CAD build for the part. Positions are in the model's coordinates, mm. Face numbers are marked on the shaded views. A direction names the side the tool comes from. Round coordinates to 2 decimals unless told otherwise and drop trailing zeros. Loops run counter-clockwise (first coordinate to the right, second up) from the corner with the lowest first, then second, coordinate; pieces in that order, holes last. Notation, with made-up numbers: M -9,27 L 5,27 A19 cw 5,41 Z; hole C 7.5,38.5 d3. An arc over 180 degrees is marked long. Use one line per item in the form item = value.
Autodesk Inventor part; units mm, degrees
ref_plane "h1_XY" through (-96.0374, 0, 0) normal (0, 1, 0) x (1, 0, 0)
ref_plane "h1_YZ" through (-96.0374, 0, 0) normal (1, 0, 0) x (0, 0, -1)
ref_plane "h1_ZX" through (-96.0374, 0, 0) normal (0, 0, -1) x (0, 1, 0)
sketch "Sketch_3" plane through (0, 0, 0) normal (0, 0, 1) x (1, 0, 0)
  line L0 (0, 0) -> (-96.0374, 0)
  line L1 (-96.0374, 0) -> (-96.0374, 1.9406)
  line L2 (-96.0374, 1.9406) -> (-95.565, 2.413)
  line L3 (-95.565, 2.413) -> (0, 2.413)
  line L4 (0, 2.413) -> (0, 0)
  line L5 (0, 0) -> (-96.0374, 0)
revolve "Revolution1" add sketch "Sketch_3" angle 360 about axis through (0, 0, 0) along (1, 0, 0)
thread "Thread1"
sketch "Sketch_17" plane through (0, 0, 0) normal (0, 0, 1) x (1, 0, 0)
  line L0 (96.0374, 0) -> (-96.0374, 0)
  line L1 (-83.5914, 2.413) -> (-83.5914, 2.159)
  line L2 (-83.5914, 2.159) -> (-83.3374, 2.159)
  line L3 (-83.3374, 2.159) -> (-83.3374, 2.413)
  line L4 (-83.3374, 2.413) -> (-83.5914, 2.413)
revolve "Revolution2" cut sketch "Sketch_17" angle 360 about axis through (96.0374, 0, 0) along (1, 0, 0)
sketch "Sketch_12" plane through (0, 0, 0) normal (0, 0, 1) x (1, 0, 0)
  line L0 (1.524, 0) -> (-15.875, 0)
  line L1 (-15.875, 0) -> (-15.875, 7.2771)
  line L2 (-15.875, 7.2771) -> (1.524, 7.2771)
  line L3 (1.524, 7.2771) -> (1.524, 0)
  line L4 (1.524, 0) -> (-15.875, 0)
revolve "Revolution3" add sketch "Sketch_12" angle 360 about axis through (1.524, 0, 0) along (1, 0, 0)
ref_plane "h1_XY" through (-96.0374, 0, 0) normal (0, 1, 0) x (1, 0, 0)
ref_plane "h1_YZ" through (-96.0374, 0, 0) normal (1, 0, 0) x (0, 0, -1)
ref_plane "h1_ZX" through (-96.0374, 0, 0) normal (0, 0, -1) x (0, 1, 0)
ref_plane "h2_XY" through (-83.3374, 0, 0) normal (0, 1, 0) x (1, 0, 0)
ref_plane "h2_YZ" through (-83.3374, 0, 0) normal (1, 0, 0) x (0, 0, -1)
ref_plane "h2_ZX" through (-83.3374, 0, 0) normal (0, 0, -1) x (0, 1, 0)
ref_plane "k1_XY" through (-96.0374, 0, -2.413) normal (0, 1, 0) x (1, 0, 0)
ref_plane "k1_YZ" through (-96.0374, 0, -2.413) normal (1, 0, 0) x (0, 0, -1)
ref_plane "k1_ZX" through (-96.0374, 0, -2.413) normal (0, 0, -1) x (0, 1, 0)
ref_plane "k2_XY" through (-96.0374, 0, 2.413) normal (0, 1, 0) x (1, 0, 0)
ref_plane "k2_YZ" through (-96.0374, 0, 2.413) normal (1, 0, 0) x (0, 0, -1)
ref_plane "k2_ZX" through (-96.0374, 0, 2.413) normal (0, 0, -1) x (0, 1, 0)
ref_plane "start_XY" through (-83.3374, 0, 0) normal (0, 1, 0) x (1, 0, 0)
ref_plane "start_YZ" through (-83.3374, 0, 0) normal (1, 0, 0) x (0, 0, -1)
ref_plane "start_ZX" through (-83.3374, 0, 0) normal (0, 0, -1) x (0, 1, 0)
ref_plane "to_prc_XY" through (-83.3374, 0, 0) normal (1, 0, 0) x (0, 0, -1)
ref_plane "to_prc_YZ" through (-83.3374, 0, 0) normal (0, 0, -1) x (0, 1, 0)
ref_plane "to_prc_ZX" through (-83.3374, 0, 0) normal (0, 1, 0) x (1, 0, 0)
ref_plane "to_rod_guide_XY" through (-96.0374, 0, 0) normal (1, 0, 0) x (0, 0, -1)
ref_plane "to_rod_guide_YZ" through (-96.0374, 0, 0) normal (0, 0, -1) x (0, 1, 0)
ref_plane "to_rod_guide_ZX" through (-96.0374, 0, 0) normal (0, 1, 0) x (1, 0, 0)
properties part number "D-75081.25-0.25XP-3.781-3pos" material "Steel"
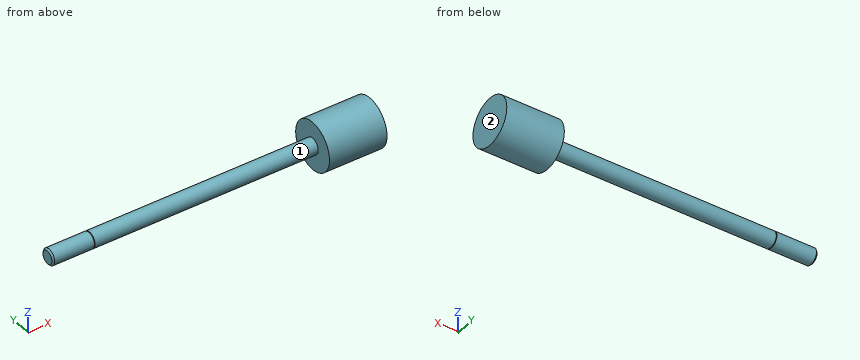
1. Cut at C-C on x = -49.5. Write the cut outline in (y, z), and give its area (3 significant figures).
Completed:
outline = C 0,0 d4.83
area = 18.3 mm2
2. Drop flat-ended pins along their axis: P1, Ø1, axis at y = -3.5, z = 4, coming from the -X side (3 decimals); P2, Ø8, axis at x = -76.5, z = 0, coming from the -Y side; P3, Ø4, axis at x = -55.5, y = -4.5, coming from the +Z side. Give the stop position or say it passes through.
Completed:
P1 = -15.875
P2 = -2.41
P3 = through
3. Probe line 1 along X through (y, z) = (-3.75, 5.25) (3 decimals); line 2 along Z through (x, y) = (-17, -0.25); line 3 along Z through (x, y) = (-54, -2). List the from-to ranges inside material, lowest first. Write a range as from..to.
Completed:
line_1 = -15.875..1.524
line_2 = -2.4..2.4
line_3 = -1.35..1.35
4. Cut at A-A on z = 0. Write the cut outline in (x, y) (3 decimals).
Completed:
outline = M -96.037,-1.941 L -95.565,-2.413 L -83.591,-2.413 L -83.591,-2.159 L -83.337,-2.159 L -83.337,-2.413 L -15.875,-2.413 L -15.875,-7.277 L 1.524,-7.277 L 1.524,7.277 L -15.875,7.277 L -15.875,2.413 L -83.337,2.413 L -83.337,2.159 L -83.591,2.159 L -83.591,2.413 L -95.565,2.413 L -96.037,1.941 Z
5. Cut at D-D on x = -5. Write the cut outline in (y, z).
Completed:
outline = C 0,0 d14.55
6. Tool access for the marked faces 1 and 2: list every direction of +Z, -Z, +X, -X, +Y, -Y with a clear straight run to the whole face (end or side of a thin tool).
Completed:
face_1 = -X
face_2 = +Z, -Z, +X, +Y, -Y
